```python
from build123d import *

# Parameters (mm, degrees)
SKETCH_1_R      = 1.45
SKETCH_1_R_2    = 1.5
SKETCH_1_R_3    = 2.5
EXTRUDE_1_DEPTH = 8
CHAMFER_1_SIZE  = 1
CHAMFER_2_SIZE  = 1


with BuildPart() as part:
    # 草图1 → 凸台-拉伸1 (new body)
    with BuildSketch(Plane.XY):
        with BuildLine():
            Line((0, 16), (-42, 16))
            ThreePointArc((-42, 16), (-46.949747468, 13.949747468), (-49, 9))
            Line((-49, 9), (-49, -16))
            Line((-49, -16), (0, -16))
            ThreePointArc((0, -16), (16, 0), (0, 16))
        make_face()
        with Locations((0, -13)):
            Circle(SKETCH_1_R, mode=Mode.SUBTRACT)
        with Locations((10.392304845, -6)):
            Circle(SKETCH_1_R_2, mode=Mode.SUBTRACT)
        with Locations((11.258330249, 6.5)):
            Circle(SKETCH_1_R, mode=Mode.SUBTRACT)
        with Locations((-10.392304845, -6)):
            Circle(SKETCH_1_R_2, mode=Mode.SUBTRACT)
        with Locations((-11.258330249, 6.5)):
            Circle(SKETCH_1_R, mode=Mode.SUBTRACT)
        with Locations((0, 12)):
            Circle(SKETCH_1_R_2, mode=Mode.SUBTRACT)
        with Locations((-42, 9)):
            Circle(SKETCH_1_R_3, mode=Mode.SUBTRACT)
        with Locations((-42, -9)):
            Circle(SKETCH_1_R_3, mode=Mode.SUBTRACT)
    extrude(amount=EXTRUDE_1_DEPTH)

    # 倒角1
    chamfer_1_edges = [part.edges().sort_by_distance(p)[0] for p in [
        (-49, -16, 4),
    ]]
    chamfer(chamfer_1_edges, length=CHAMFER_1_SIZE)

    # 倒角2
    # the kernel refuses this chamfer: 1 mm, written as the material it takes off along each edge
    with BuildSketch(Plane(origin=(-50.571682988, -16, 8), x_dir=(0, 0.9996219169112968, 0.027495876610585647), z_dir=(1, 0, 0))) as chamfer_2_piece_1:
        Polygon((CHAMFER_2_SIZE * 0.999621916911, -CHAMFER_2_SIZE * 0.0274958766106), (-CHAMFER_2_SIZE * 0.0274958766106, -CHAMFER_2_SIZE * 0.999621916911), (0, 0), align=None)
    extrude(amount=50.571682988, mode=Mode.SUBTRACT)
    with BuildSketch(Plane(origin=(-49, 9, 8), x_dir=(-0.02749587661058907, 0, -0.9996219169112965), z_dir=(0, -1, 0))) as chamfer_2_piece_2:
        Polygon((CHAMFER_2_SIZE * 0.999621916911, CHAMFER_2_SIZE * 0.0274958766106), (-CHAMFER_2_SIZE * 0.0274958766106, CHAMFER_2_SIZE * 0.999621916911), (0, 0), align=None)
    extrude(amount=26.571682988, mode=Mode.SUBTRACT)
    with BuildSketch(Plane(origin=(0, 0, 8), x_dir=(0, -1, 0), z_dir=(-1, 0, 0))) as chamfer_2_piece_3:
        Polygon((16 - CHAMFER_2_SIZE, 0), (16, -CHAMFER_2_SIZE), (16, 0), align=None)
    revolve(axis=Axis((0, 0, 8), (0, 0, 1)), revolution_arc=180, mode=Mode.SUBTRACT)
    with BuildSketch(Plane(origin=(-42, 9, 8), x_dir=(0, 1, 0), z_dir=(1, 0, 0))) as chamfer_2_piece_4:
        Polygon((7, -CHAMFER_2_SIZE), (7 - CHAMFER_2_SIZE, 0), (7, 0), align=None)
    revolve(axis=Axis((-42, 9, 8), (0, 0, 1)), revolution_arc=90, mode=Mode.SUBTRACT)
    with BuildSketch(Plane(origin=(0, 16, 8), x_dir=(0, -0.9996219169112968, 0.027495876610585647), z_dir=(-1, 0, 0))) as chamfer_2_piece_5:
        Polygon((CHAMFER_2_SIZE * 0.999621916911, -CHAMFER_2_SIZE * 0.0274958766106), (-CHAMFER_2_SIZE * 0.0274958766106, -CHAMFER_2_SIZE * 0.999621916911), (0, 0), align=None)
    extrude(amount=42, mode=Mode.SUBTRACT)


solid = part.part
```
Verification items for the finished model (mm, model axes). Give positions to 0.01 mm unless a question says otherwise; leave off trailing zeros.
1. Mould release check, pull along X, two halves, no side actions. Record for faces 1 (the cylindrical face through (-11.89, -5.93, 3.94)), 2 (the conical face through (-46.31, 13.4, 7.84)), 3 (the conical face through (15.17, -0.334, 7.826)): released by +X, released by -X, zero draft, split by the parting line, or undercut.
2. Thickness scan on line 1 (Y direction, x = -42, z = 5.5); line 2 (Y direction, x = -44, z = 4); line 3 (X direction, y = 5.5, z = 4). Record the ranges inside material, lowest first.
3. Go/stop test with a flat-tipped pin: pin 1 Ø3.5 at (x, y) = (-10.39, -6) entering from +Z. Record where the tip stops, or that it passes through.
4. Section check A-A, the plane z = 4. Count the separate pieces of the cut face and the enclosed holes in it, then the cut area to 3 significant figures.
Geometry says:
1. face 1: undercut
1. face 2: released by -X
1. face 3: released by +X
2. line 1: y = -16 to -11.5, -6.5 to 6.5, 11.5 to 16
2. line 2: y = -16 to -10.5, -7.5 to 7.5, 10.5 to 15.71
2. line 3: x = -49 to -12.31, -10.21 to 10.21, 12.31 to 15.02
3. pin 1: stops at z = 8
4. separate pieces: 1
4. enclosed holes: 8
4. area: 1,880 mm2
